Here's how the part is built. I have some questions about the finished solid (model axes, mm). Face numbers are marked on the shaded views. A direction names the side the tool comes from. Give positions to 0.01 mm unless a question says otherwise; leave off trailing zeros. Loops run counter-clockwise (first coordinate to the right, second up) from the corner with the lowest first, then second, coordinate; pieces in that order, holes last. Notation, with made-up numbers: (28, -1) - (38, -1) arc R20 cw to (38, 4) - close; hole circle Ø9 at (-26, 45.5). An arc over 180 degrees is marked (long way). Return JSON: item names as keys, results as strings. Group by question number.
(1) On a 3-axis mill with a long thin cutter (end or side, diameter ignored), from which of +Z, -Z, +X, -X, +Y, -Y can I reach the whole of each face in a straight line? I mean the marked faces 4, 5, 6 and 7. Say none if no direction works.
(2) If we section it at A-A (z = 5.5): Please give me the cut outline in (x, y).
(3) If we section it at D-D (z = 2.5): Please give me the cut outline in (x, y).
(4) I need wall thicknesses on probe 1 along Z at (x, y) = (-10.5, 9.25); probe 2 along X at (y, z) = (-13, 12.25). Which ranges of each line are inside material? Lowest first, please. Write a range as [from, to].
(5) If we section it at B-B (y = 0): Please give me the cut outline in (x, z).
(6) If we mould it in two halves opening along Z, with no side actions, what happens to the marked faces 1, 2 and 3? For each: released by +Z, released by -Z, zero draft, split by the parting line, or undercut.
(7) For P1, Ø1.1, axis at y = 0, z = 11, coming from the -X side; P2, Ø1, axis at x = 9.5, z = 7, coming from the -Y side; P3, Ø1.1, axis at y = 0, z = 9.5, coming from the +X side, each with a flat end and sliding along its axis, tell me the tip position at first contact or that it passes through.
```python
from build123d import *

# Parameters (mm, degrees)
CYLINDER005_R               = 12
CYLINDER005_DEPTH           = 20
CYLINDER006_R               = 15
CYLINDER006_DEPTH           = 3.5
CYLINDER007_R               = 15
CYLINDER007_DEPTH           = 1.5
CYLINDER008_R               = 15
CYLINDER008_DEPTH           = 1.5
CYLINDER009_R               = 15
CYLINDER009_DEPTH           = 3.5
BOX002_W                    = 29
BOX002_H                    = 1
BOX002_DEPTH                = 10
BOX003_W                    = 29
BOX003_H                    = 1
BOX003_DEPTH                = 10
COMPOUND001_PLACEMENT_ANGLE = 90


with BuildPart() as cylinder005:
    # Cylinder005 → Cylinder005 (new body)
    with BuildSketch(Plane.XY):
        Circle(CYLINDER005_R)
    extrude(amount=CYLINDER005_DEPTH)


with BuildPart() as cylinder006:
    # Cylinder006 → Cylinder006 (new body)
    with BuildSketch(Plane.XY):
        Circle(CYLINDER006_R)
    extrude(amount=CYLINDER006_DEPTH)


with BuildPart() as cylinder007:
    # Cylinder007 → Cylinder007 (new body)
    with BuildSketch(Plane.XY.offset(3.5)):
        Circle(CYLINDER007_R)
    extrude(amount=CYLINDER007_DEPTH)


with BuildPart() as cylinder008:
    # Cylinder008 → Cylinder008 (new body)
    with BuildSketch(Plane.XY.offset(18.5)):
        Circle(CYLINDER008_R)
    extrude(amount=CYLINDER008_DEPTH)


with BuildPart() as cylinder009:
    # Cylinder009 → Cylinder009 (new body)
    with BuildSketch(Plane.XY.offset(15)):
        Circle(CYLINDER009_R)
    extrude(amount=CYLINDER009_DEPTH)


with BuildPart() as cube002:
    # Box002 → Box002 (new body)
    with BuildSketch(Plane(origin=(-14.5, -0.5, 5), x_dir=(1, 0, 0), z_dir=(0, 0, 1))):
        with Locations((14.5, 0.5)):
            Rectangle(BOX002_W, BOX002_H)
    extrude(amount=BOX002_DEPTH)


with BuildPart() as basewheel_filledsides:
    # Box003 → Box003 (new body)
    with BuildSketch(Plane(origin=(-14.5, -0.5, 5), x_dir=(1, 0, 0), z_dir=(0, 0, 1))):
        with Locations((14.5, 0.5)):
            Rectangle(BOX003_W, BOX003_H)
    extrude(amount=BOX003_DEPTH)


with BuildPart() as basewheel_filledsides_1:
    # Compound001 placement: moved
    add(basewheel_filledsides.part.rotate(Axis((0, 0, 0), (0, 0, 1)), COMPOUND001_PLACEMENT_ANGLE))

    # Fusion001: union Cylinder005, Cylinder006, Cylinder007, Cylinder008, Cylinder009, Cube002
    add(cylinder005.part)
    add(cylinder006.part)
    add(cylinder007.part)
    add(cylinder008.part)
    add(cylinder009.part)
    add(cube002.part)


solid = basewheel_filledsides_1.part
```
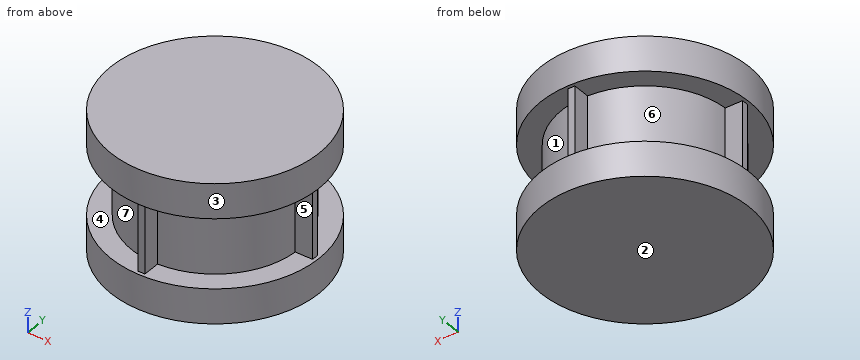
Values:
{
 "1": {"face 4": "none", "face 5": "+X, -Y", "face 6": "-X, +Y", "face 7": "-X, -Y"},
 "2": {"outline": "(-14.5, -0.5) - (-11.99, -0.5) arc R12 ccw to (-0.5, -11.99) - (-0.5, -14.5) - (0.5, -14.5) - (0.5, -11.99) arc R12 ccw to (11.99, -0.5) - (14.5, -0.5) - (14.5, 0.5) - (11.99, 0.5) arc R12 ccw to (0.5, 11.99) - (0.5, 14.5) - (-0.5, 14.5) - (-0.5, 11.99) arc R12 ccw to (-11.99, 0.5) - (-14.5, 0.5) - close"},
 "3": {"outline": "circle Ø30 at (0, 0)"},
 "4": {"probe 1": "[0, 5], [15, 20]", "probe 2": "[-0.5, 0.5]"},
 "5": {"outline": "(-15, 0) - (15, 0) - (15, 5) - (14.5, 5) - (14.5, 15) - (15, 15) - (15, 20) - (-15, 20) - (-15, 15) - (-14.5, 15) - (-14.5, 5) - (-15, 5) - close"},
 "6": {"face 1": "undercut", "face 2": "released by -Z", "face 3": "zero draft"},
 "7": {"P1": "x = -14.5", "P2": "y = -7.94", "P3": "x = 14.5"}
}
